```python
from build123d import *

# Parameters (mm, degrees)
F0_W      = 447.7258
F0_H      = 987.425
F1_DEPTH  = 19.05
F3_D      = 8.001
F3_DEPTH  = 25.4
F3_TIP    = 2.4037429064
F4_R      = 30.1625
F5_DEPTH  = 25.4
F6_D      = 15.0114
F6_DEPTH  = 14.224
F6_TIP    = 4.5098795482
F8_D      = 8.001
F8_DEPTH  = 25.4
F8_TIP    = 2.4037429064
F10_D     = 8.001
F10_DEPTH = 25.4
F10_TIP   = 2.4037429064
F12_D     = 8.001
F12_DEPTH = 25.4
F12_TIP   = 2.4037429064
F13_D     = 3.175
F13_DEPTH = 25.4
F13_TIP   = 0.9538662327


with BuildPart() as f1:
    # F0 (on Front) → F1 (new body)
    with BuildSketch(Plane.XZ):
        Rectangle(F0_W, F0_H)
    extrude(amount=F1_DEPTH)

    # F3
    with Locations(Plane.XZ.offset(19.05)):
        with Locations((-214.3379, 442.9125), (-214.3379, 0), (-214.3379, -442.9125)):
            Hole(F3_D / 2, depth=F3_DEPTH)
            with Locations((0, 0, -(F3_DEPTH + F3_TIP / 2))):  # 118° drill point
                Cone(0, F3_D / 2, F3_TIP, mode=Mode.SUBTRACT)

    # F4 (on face) → F5 (cut)
    with BuildSketch(Plane.XZ.offset(19.05)):
        with Locations((20.6629, 0)):
            Circle(F4_R)
    extrude(amount=-F5_DEPTH, mode=Mode.SUBTRACT)

    # F6
    with Locations(Plane.XZ.offset(19.05)):
        with Locations((-173.0629, 469.8365), (0, 469.8365), (173.0629, 469.8365), (199.9869, 442.9125), (199.9869, 0), (199.9869, -442.9125), (173.0629, -469.8365), (0, -469.8365), (-173.0629, -469.8365)):
            Hole(F6_D / 2, depth=F6_DEPTH)
            with Locations((0, 0, -(F6_DEPTH + F6_TIP / 2))):  # 118° drill point
                Cone(0, F6_D / 2, F6_TIP, mode=Mode.SUBTRACT)

    # F8
    with Locations(Plane(origin=(0, 0, -493.7125), x_dir=(1, 0, 0), z_dir=(0, 0, -1))):
        with Locations((-173.0629, 9.525), (0, 9.525), (173.0629, 9.525)):
            Hole(F8_D / 2, depth=F8_DEPTH)
            with Locations((0, 0, -(F8_DEPTH + F8_TIP / 2))):  # 118° drill point
                Cone(0, F8_D / 2, F8_TIP, mode=Mode.SUBTRACT)

    # F10
    with Locations(Plane.XY.offset(493.7125)):
        with Locations((-173.0629, -9.525), (0, -9.525), (173.0629, -9.525)):
            Hole(F10_D / 2, depth=F10_DEPTH)
            with Locations((0, 0, -(F10_DEPTH + F10_TIP / 2))):  # 118° drill point
                Cone(0, F10_D / 2, F10_TIP, mode=Mode.SUBTRACT)

    # F12
    with Locations(Plane.YZ.offset(223.8629)):
        with Locations((-9.525, 0), (-9.525, -442.9125), (-9.525, 442.9125)):
            Hole(F12_D / 2, depth=F12_DEPTH)
            with Locations((0, 0, -(F12_DEPTH + F12_TIP / 2))):  # 118° drill point
                Cone(0, F12_D / 2, F12_TIP, mode=Mode.SUBTRACT)

    # F13
    with Locations(Plane.XZ.offset(19.05)):
        with Locations((-214.3379, 392.1125), (-214.3379, 203.2), (-214.3379, -203.2), (-214.3379, -392.1125)):
            Hole(F13_D / 2, depth=F13_DEPTH)
            with Locations((0, 0, -(F13_DEPTH + F13_TIP / 2))):  # 118° drill point
                Cone(0, F13_D / 2, F13_TIP, mode=Mode.SUBTRACT)


solid = f1.part
```
Check sheet for the modelled part. Datum: model origin and axes. Units: mm. Give positions to 0.01 mm unless a question says otherwise; leave off trailing zeros. Write each loop counter-clockwise with the first axis right and the second up, starting at its lowest first coordinate (ties: lowest second). Pieces come first, ordered by that corner, then holes.
Item 1: Cross-section at A-A (x = 31). Enter the section's corners in (y, z), and give its area (3 significant figures).
Item 2: Gauge pin test, flat ends, axial feed: pin 1 (7 mm diameter, centred on x = -214.34, z = 0, fed in from -Y); pin 2 (6.5 mm diameter, centred on x = 173.06, y = -9.52, fed in from -Z); pin 3 (12 mm diameter, centred on x = 199.99, z = 0, fed in from -Y); pin 4 (6.5 mm diameter, centred on x = -173.06, y = -9.52, fed in from +Z). Record the tip position at first contact, or that the pin passes through.
Item 3: Scan lines: L1, parallel to Z at x = 198.5, y = -5.5; L2, parallel to Z at x = -167, y = -6.5; L3, parallel to X at y = -10, z = -203.2. Record each from-to range of solid material in increasing order.
Item 4: Draft check along X on faces 1 (the face through (-53, 0, 7)), 2 (the face through (49.433, -9.658, 9.06)), 3 (the face through (-223.863, -9, -7)). Enter one of: released by +X, released by -X, zero draft, split by the parting line, or undercut.
Report:
1. outline: (-19.05, -493.71) - (0, -493.71) - (0, -28.34) - (-19.05, -28.34) - close; (-19.05, 28.34) - (0, 28.34) - (0, 493.71) - (-19.05, 493.71) - close
1. area: 17,700 mm2
2. pin 1: passes through
2. pin 2: stops at z = -463.07
2. pin 3: stops at y = -3.92
2. pin 4: stops at z = 463.07
3. L1: z = -493.71 to -450.27, -435.56 to -7.36, 7.36 to 435.56, 450.27 to 493.71
3. L2: z = -493.71 to -474.26, -465.41 to 465.41, 474.26 to 493.71
3. L3: x = -223.86 to -215.93, -212.75 to 223.86
4. face 1: zero draft
4. face 2: undercut
4. face 3: released by -X
